from build123d import *

# Parameters (mm, degrees)
SKETCH1_W           = 56
SKETCH1_H           = 40
SKETCH1_W_2         = 36
SKETCH1_H_2         = 30
BOSS_EXTRUDE1_DEPTH = 1.5
SKETCH2_W           = 54
SKETCH2_H           = 38
SKETCH2_W_2         = 44.5
SKETCH2_H_2         = 34.5
BOSS_EXTRUDE2_DEPTH = 3
SKETCH3_W           = 10
SKETCH3_H           = 1.75
BOSS_EXTRUDE3_DEPTH = 16
SKETCH4_W           = 10
SKETCH4_H           = 4
BOSS_EXTRUDE4_DEPTH = 4
SKETCH6_W           = 10
SKETCH6_H           = 4
BOSS_EXTRUDE5_DEPTH = 4
CHAMFER1_SIZE       = 4
SKETCH7_R           = 1.25
CUT_EXTRUDE2_DEPTH  = 6
FILLET1_R           = 1


with BuildPart() as part:
    # Sketch1 → Boss-Extrude1 (new body)
    with BuildSketch(Plane.XY):
        Rectangle(SKETCH1_W, SKETCH1_H)
        Rectangle(SKETCH1_W_2, SKETCH1_H_2, mode=Mode.SUBTRACT)
    extrude(amount=BOSS_EXTRUDE1_DEPTH)

    # Sketch2 → Boss-Extrude2 (add)
    with BuildSketch(Plane.XY.offset(1.5)):
        Rectangle(SKETCH2_W, SKETCH2_H)
        with Locations((3, 0)):
            Rectangle(SKETCH2_W_2, SKETCH2_H_2, mode=Mode.SUBTRACT)
    extrude(amount=BOSS_EXTRUDE2_DEPTH)

    # Sketch3 → Boss-Extrude3 (add)
    with BuildSketch(Plane.XY.offset(4.5)):
        with Locations((0, 18.125)):
            Rectangle(SKETCH3_W, SKETCH3_H)
        with Locations((0, -18.125)):
            Rectangle(SKETCH3_W, SKETCH3_H)
    extrude(amount=BOSS_EXTRUDE3_DEPTH)

    # Sketch4 → Boss-Extrude4 (add)
    with BuildSketch(Plane(origin=(0, 17.25, 0), x_dir=(-1, 0, 0), z_dir=(0, -1, 0))):
        with Locations((0, -18.5)):
            Rectangle(SKETCH4_W, SKETCH4_H)
    extrude(amount=BOSS_EXTRUDE4_DEPTH)

    # Sketch6 → Boss-Extrude5 (add)
    with BuildSketch(Plane(origin=(0, -17.25, 0), x_dir=(1, 0, 0), z_dir=(0, 1, 0))):
        with Locations((0, -18.5)):
            Rectangle(SKETCH6_W, SKETCH6_H)
    extrude(amount=BOSS_EXTRUDE5_DEPTH)

    # Chamfer1
    chamfer1_edges = [part.edges().sort_by_distance(p)[0] for p in [
        (0, -17.25, 16.5),
        (0, 17.25, 16.5),
    ]]
    chamfer(chamfer1_edges, length=CHAMFER1_SIZE - 0.0001)  # a hair under: the kernel refuses the full size

    # Sketch7 → Cut-Extrude2 (cut)
    with BuildSketch(Plane.XY.offset(20.5)):
        with Locations((0, 16.125)):
            Circle(SKETCH7_R)
        with Locations((0, -16.125)):
            Circle(SKETCH7_R)
    extrude(amount=-CUT_EXTRUDE2_DEPTH, mode=Mode.SUBTRACT)

    # Fillet1
    fillet1_edges = [part.edges().sort_by_distance(p)[0] for p in [
        (-27, 19, 3),
        (-27, -19, 3),
        (27, -19, 3),
        (27, 19, 3),
        (-28, 20, 0.75),
        (28, 20, 0.75),
        (28, -20, 0.75),
        (-28, -20, 0.75),
    ]]
    fillet(fillet1_edges, radius=FILLET1_R)


solid = part.part
Source: CAD feature listing. Evaluate the final solid. Frame: model axes, mm. A direction names the side the tool comes from. Give positions to 0.01 mm unless a question says otherwise; leave off trailing zeros. Loops run counter-clockwise (first coordinate to the right, second up) from the corner with the lowest first, then second, coordinate; pieces in that order, holes last. Notation, with made-up numbers: (68, 68) -> (78, 68) arc R23 ccw to (78, 76) -> close; hole circle Ø10 at (21.5, 39.5). An arc over 180 degrees is marked (long way). Use a Markdown table: item, result. Add a question column.
1) Pull-direction query (Z, two-part tool) for faces 4 (the face through (0, 16, 14.5)), 5 (the face through (0, -13.25, 18)), 6 (the face through (3, 17.25, 4)); classes: +Z half, -Z half, draft (parallel to the pull), parting line (faces both ways), or undercut.
2) Reachability of faces 1 (the face through (0, -15, 1)), 2 (the face through (0, 19, 7)), 3 (the face through (-5, 17, 14)) from +Z, -Z, +X, -X, +Y, -Y: full face, straight path, thin tool, end or side. Return the list, or none.
3) Section query A-A, the plane y = -9. Return the cut outline in (x, z), then the cut area to 3 significant figures.
4) Section query C-C, the plane z = 10.25. Return the cut outline in (x, y).
5) First-contact query: pin 1 (5.5 mm diameter, centred on x = -3, z = 6.5, fed in from -Y); pin 2 (6.5 mm diameter, centred on y = 15, z = 10, fed in from +X); pin 3 (5 mm diameter, centred on x = -8.5, z = 15.5, fed in from -Y); pin 4 (3 mm diameter, centred on x = -1.5, z = 19, fed in from +Y). Flat tips, straight axial feed; report the tip coordinate or a pass-through.
6) Line query: line 1 along Y through (x, z) = (0, 18.15) (3 decimals); line 2 along Y through (x, z) = (0, 16.4) (3 decimals); line 3 along Z through (x, y) = (7, 16). Output: solid intervals per line, ascending. Write a range as [from, to].
7) Section query D-D, the plane x = 20. Return the cut outline in (y, z).
8) Section query B-B, the plane x = -11. Return the cut outline in (y, z).
Numbers:
| question | item | result |
|---|---|---|
| 1 | face 4 | +Z half |
| 1 | face 5 | draft |
| 1 | face 6 | undercut |
| 2 | face 1 | -Z |
| 2 | face 2 | +Z, +X, -X, +Y |
| 2 | face 3 | +Z, -X, +Y, -Y |
| 3 | outline | (-28, 0) -> (-18, 0) -> (-18, 1.5) -> (-19.25, 1.5) -> (-19.25, 4.5) -> (-27, 4.5) -> (-27, 1.5) -> (-28, 1.5) -> close; (18, 0) -> (28, 0) -> (28, 1.5) -> (27, 1.5) -> (27, 4.5) -> (25.25, 4.5) -> (25.25, 1.5) -> (18, 1.5) -> close |
| 3 | area | 58.5 mm2 |
| 4 | outline | (-5, -19) -> (5, -19) -> (5, -17.25) -> (-5, -17.25) -> close; (-5, 17.25) -> (5, 17.25) -> (5, 19) -> (-5, 19) -> close |
| 5 | pin 1 | stops at y = -19 |
| 5 | pin 2 | stops at x = 5 |
| 5 | pin 3 | passes through |
| 5 | pin 4 | stops at y = 19 |
| 6 | line 1 | y = [-19, -17.375], [-14.875, -13.25], [13.25, 14.875], [17.375, 19] |
| 6 | line 2 | y = [-19, -17.375], [-14.875, -13.35], [13.35, 14.875], [17.375, 19] |
| 6 | line 3 | z = [0, 1.5] |
| 7 | outline | (-20, 0) -> (20, 0) -> (20, 1.5) -> (19, 1.5) -> (19, 4.5) -> (17.25, 4.5) -> (17.25, 1.5) -> (-17.25, 1.5) -> (-17.25, 4.5) -> (-19, 4.5) -> (-19, 1.5) -> (-20, 1.5) -> close |
| 8 | outline | (-20, 0) -> (-15, 0) -> (-15, 1.5) -> (-17.25, 1.5) -> (-17.25, 4.5) -> (-19, 4.5) -> (-19, 1.5) -> (-20, 1.5) -> close; (15, 0) -> (20, 0) -> (20, 1.5) -> (19, 1.5) -> (19, 4.5) -> (17.25, 4.5) -> (17.25, 1.5) -> (15, 1.5) -> close |
